```python
from build123d import *

# Parameters (mm, degrees)
SKETCH1_R           = 8.5
BOSS_EXTRUDE1_DEPTH = 1.9
BOSS_EXTRUDE2_DEPTH = 1.9
CIRPATTERN2_COUNT   = 12
FILLET5_R           = 6
FILLET6_R           = 6
BOSS_EXTRUDE3_DEPTH = 1.9
SKETCH6_W           = 11.017873235
SKETCH6_H           = 24.192230011
CUT_EXTRUDE2_DEPTH  = 24.342236397
SKETCH8_R           = 5
BOSS_EXTRUDE4_DEPTH = 3
SKETCH14_W          = 5
SKETCH14_H          = 10
BOSS_EXTRUDE8_DEPTH = 3
SKETCH17_R          = 1.5
CUT_EXTRUDE10_DEPTH = 24.342236397
FILLET9_R           = 2.5
FILLET10_R          = 2.5
CUT_EXTRUDE11_DEPTH = 2
SKETCH20_R          = 3.6
CUT_EXTRUDE12_DEPTH = 24.457408211


# Some blends are built 0.0001 mm under size
with BuildPart() as part:
    # Sketch1 → Boss-Extrude1 (new body)
    with BuildSketch(Plane.XY):
        with Locations(Location((0, 0, 0), (0, 0, 180))):
            Circle(SKETCH1_R)
    extrude(amount=BOSS_EXTRUDE1_DEPTH)

    # Sketch3 → Boss-Extrude2 (add)
    with BuildSketch(Plane.XY.offset(1.9)):
        Polygon((-1.305261922, 9.914448614), (-1.509060022, 7), (1.509060022, 7), (1.305261922, 9.914448614), (0.678518537, 11), (-0.678518537, 11), align=None)
    boss_extrude2 = extrude(amount=-BOSS_EXTRUDE2_DEPTH)

    # CirPattern2: Boss-Extrude2 ×12 about axis
    cirpattern2_axis = Axis((0, 0, 0), (0, 0, 1))
    for i in range(1, CIRPATTERN2_COUNT):
        add(boss_extrude2.rotate(cirpattern2_axis, i * 360 / CIRPATTERN2_COUNT))

    # Fillet5
    # the kernel refuses this fillet: 6 mm, written as the material it takes off along each edge
    with BuildSketch(Plane(origin=(9.238795325, 3.826834324, 5.354382408), x_dir=(0.49999999999981276, 0.8660254037845467, 0), z_dir=(0, 0, -1)), Plane(origin=(1.305261922, 9.914448614, 5.354382408), x_dir=(-0.5000000000001841, 0.8660254037843323, 0), z_dir=(0, 0, -1)), Plane(origin=(-7.933533403, 6.08761429, 5.354382408), x_dir=(-1, 0, 0), z_dir=(0, 0, -1)), Plane(origin=(-9.914448614, 1.305261922, 5.354382408), x_dir=(-0.8660254037843321, -0.5000000000001844, 0), z_dir=(0, 0, -1)), Plane(origin=(-9.238795325, -3.826834324, 5.354382408), x_dir=(-0.49999999999981826, -0.8660254037845436, 0), z_dir=(0, 0, -1)), Plane(origin=(-6.08761429, -7.933533403, 5.354382408), x_dir=(0, -1, 0), z_dir=(0, 0, -1)), Plane(origin=(3.826834324, -9.238795325, 5.354382408), x_dir=(0.8660254037845474, -0.49999999999981154, 0), z_dir=(0, 0, -1)), Plane(origin=(7.933533403, -6.08761429, 5.354382408), x_dir=(1, 0, 0), z_dir=(0, 0, -1)), Plane(origin=(9.914448614, -1.305261922, 5.354382408), x_dir=(0.866025403784333, 0.500000000000183, 0), z_dir=(0, 0, -1))) as fillet5_piece_1:
        with BuildLine():
            CenterArc((1.388315544, -5.998484909), FILLET5_R, 91.287628333, 24.712371667)
            Line((-1.241911337, -0.605720631), (-1.294515874, -0.497865346))
            Line((-1.294515874, -0.497865346), (-0.052604538, 0.107855286))
            Line((-0.052604538, 0.107855286), (0, 0.12))
            ThreePointArc((0, 0.12), (0.626743385, 0.12), (1.250790195, 0.119969698))
            Line((1.250790195, 0.119969698), (1.25348677, 0))
        make_face()
    extrude(amount=8.808764816, mode=Mode.SUBTRACT)
    with BuildSketch(Plane(origin=(6.08761429, 7.933533403, 5.354382408), x_dir=(-0.4383711467890806, -0.8987940462991654, 0), z_dir=(0, 0, -1)), Plane(origin=(-3.826834324, 9.238795325, 5.354382408), x_dir=(0.5591929034707432, -0.8290375725550441, 0), z_dir=(0, 0, -1)), Plane(origin=(-1.305261922, -9.914448614, 5.354382408), x_dir=(-0.06975647374412203, 0.9975640502598244, 0), z_dir=(0, 0, -1))) as fillet5_piece_2:
        with BuildLine():
            CenterArc((1.381752963, 6), FILLET5_R, 245.287628333, 24.712371667)
            Line((-1.126626446, 0.549492433), (-1.176794034, 0.440482282))
            ThreePointArc((-1.176794034, 0.440482282), (-0.615917761, 0.166890931), (-0.052604538, -0.107855286))
            Line((-0.052604538, -0.107855286), (0, -0.12))
            Line((0, -0.12), (1.381752963, -0.12))
            Line((1.381752963, -0.12), (1.381752963, 0))
        make_face()
    extrude(amount=8.808764816, mode=Mode.SUBTRACT)

    # Fillet6
    # the kernel refuses this fillet: 6 mm, written as the material it takes off along each edge
    with BuildSketch(Plane(origin=(7.933533403, 6.08761429, 5.354382408), x_dir=(-0.8987940462991681, -0.4383711467890751, 0), z_dir=(0, 0, -1)), Plane(origin=(3.826834324, 9.238795325, 5.354382408), x_dir=(-0.5591929034707512, -0.8290375725550386, 0), z_dir=(0, 0, -1)), Plane(origin=(-1.305261922, 9.914448614, 5.354382408), x_dir=(-0.06975647374412959, -0.9975640502598239, 0), z_dir=(0, 0, -1)), Plane(origin=(-6.08761429, 7.933533403, 5.354382408), x_dir=(0.43837114678907496, -0.8987940462991681, 0), z_dir=(0, 0, -1)), Plane(origin=(-9.238795325, 3.826834324, 5.354382408), x_dir=(0.8290375725550395, -0.5591929034707501, 0), z_dir=(0, 0, -1)), Plane(origin=(-9.914448614, -1.305261922, 5.354382408), x_dir=(0.9975640502598241, -0.0697564737441288, 0), z_dir=(0, 0, -1)), Plane(origin=(-7.933533403, -6.08761429, 5.354382408), x_dir=(0.8987940462991686, 0.4383711467890744, 0), z_dir=(0, 0, -1)), Plane(origin=(-3.826834324, -9.238795325, 5.354382408), x_dir=(0.5591929034707488, 0.8290375725550403, 0), z_dir=(0, 0, -1)), Plane(origin=(1.305261922, -9.914448614, 5.354382408), x_dir=(0.06975647374412966, 0.9975640502598239, 0), z_dir=(0, 0, -1)), Plane(origin=(6.08761429, -7.933533403, 5.354382408), x_dir=(-0.4383711467890749, 0.8987940462991683, 0), z_dir=(0, 0, -1)), Plane(origin=(9.238795325, -3.826834324, 5.354382408), x_dir=(-0.8290375725550393, 0.5591929034707505, 0), z_dir=(0, 0, -1)), Plane(origin=(9.914448614, 1.305261922, 5.354382408), x_dir=(-0.9975640502598239, 0.06975647374412894, 0), z_dir=(0, 0, -1))) as fillet6_piece_1:
        with BuildLine():
            CenterArc((1.381752963, -6), FILLET6_R, 90, 24.712371667)
            Line((-1.126626446, -0.549492433), (-1.176794034, -0.440482282))
            ThreePointArc((-1.176794034, -0.440482282), (-0.615917761, -0.166890931), (-0.052604538, 0.107855286))
            Line((-0.052604538, 0.107855286), (0, 0.12))
            Line((0, 0.12), (1.381752963, 0.12))
            Line((1.381752963, 0.12), (1.381752963, 0))
        make_face()
    extrude(amount=8.808764816, mode=Mode.SUBTRACT)

    # Sketch4 → Boss-Extrude3 (add)
    with BuildSketch(Plane(origin=(0, 0, 0), x_dir=(-1, 0, 0), z_dir=(0, 0, -1))):
        with BuildLine():
            Line((-2.5, 20.5), (-2.5, 4.330127019))
            ThreePointArc((-2.5, 4.330127019), (-5, 0), (-2.5, -4.330127019))
            Line((-2.5, -4.330127019), (-2.5, -11))
            Line((-2.5, -11), (2.5, -11))
            Line((2.5, -11), (2.5, -4.330127019))
            ThreePointArc((2.5, -4.330127019), (5, 0), (2.5, 4.330127019))
            Line((2.5, 4.330127019), (2.5, 20.5))
            Line((2.5, 20.5), (-2.5, 20.5))
        make_face()
    extrude(amount=-BOSS_EXTRUDE3_DEPTH)

    # Sketch6 → Cut-Extrude2 (cut, through all)
    with BuildSketch(Plane(origin=(0, 0, 0), x_dir=(-1, 0, 0), z_dir=(0, 0, -1))):
        with Locations((-8.008936618, 1.096115006)):
            Rectangle(SKETCH6_W, SKETCH6_H)
    extrude(amount=-CUT_EXTRUDE2_DEPTH, mode=Mode.SUBTRACT)

    # Sketch8 → Boss-Extrude4 (add)
    with BuildSketch(Plane(origin=(0, 0, 0), x_dir=(-1, 0, 0), z_dir=(0, 0, -1))):
        Circle(SKETCH8_R)
    extrude(amount=-BOSS_EXTRUDE4_DEPTH)

    # Sketch14 → Boss-Extrude8 (add)
    with BuildSketch(Plane(origin=(0, 0, 0), x_dir=(-1, 0, 0), z_dir=(0, 0, -1))):
        with Locations((2.5, 0)):
            Rectangle(SKETCH14_W, SKETCH14_H)
    extrude(amount=-BOSS_EXTRUDE8_DEPTH)

    # Sketch17 → Cut-Extrude10 (cut, through all)
    with BuildSketch(Plane.XY.offset(1.9)):
        with Locations((0, 18)):
            Circle(SKETCH17_R)
    extrude(amount=-CUT_EXTRUDE10_DEPTH, mode=Mode.SUBTRACT)

    # Fillet9
    fillet9_edges = [part.edges().sort_by_distance(p)[0] for p in [
        (-2.5, 20.5, 0.95),
        (2.5, 20.5, 0.95),
    ]]
    fillet(fillet9_edges, radius=FILLET9_R - 0.0001)  # a hair under: the kernel refuses the full size

    # Fillet10
    fillet10_edges = [part.edges().sort_by_distance(p)[0] for p in [
        (2.5, -11, 0.95),
    ]]
    fillet(fillet10_edges, radius=FILLET10_R)

    # Sketch19 → Cut-Extrude11 (cut)
    with BuildSketch(Plane.XY.offset(3)):
        Polygon((0, 3.6), (-5.102940329, 2.6), (-5.102940329, -2.6), (0, -3.6), align=None)
    extrude(amount=-CUT_EXTRUDE11_DEPTH, mode=Mode.SUBTRACT)

    # Sketch20 → Cut-Extrude12 (cut, through all)
    with BuildSketch(Plane.XY.offset(3)):
        Circle(SKETCH20_R)
    extrude(amount=-CUT_EXTRUDE12_DEPTH, mode=Mode.SUBTRACT)


solid = part.part
```
Geometry check sheet. Reference: the model listing, model coordinates, mm. A direction names the side the tool comes from. Round coordinates to 2 decimals unless told otherwise and drop trailing zeros. Order: outer loops, then holes, each group sorted by start corner. A loop starts at its lowest first (then second) coordinate and runs counter-clockwise, first axis right, second up. Notation, with made-up numbers: M 27,-7.75 L 35,-7.75 A21 ccw 35,15.25 Z; hole C -29,55 d6. An arc over 180 degrees is marked long. Write item = value, one per line.
Q1. Section check C-C (z = 0.6). Give the number of separate pieces and of enclosed holes in the cut face, plus the area to 3 significant figures.
Answer block:
separate_pieces = 1
enclosed_holes = 2
area = 222 mm^2
Q2. Section check D-D (x = -4.5). Enter the section's corners in (y, z).
Answer block:
outline = M -9.59,0 L 9.59,0 L 9.59,1.9 L 5,1.9 L 5,3 L 2.72,3 L 2.72,1 L -2.72,1 L -2.72,3 L -5,3 L -5,1.9 L -9.59,1.9 Z
Q3. Scan lines: line 1 (Y direction, x = 0, z = 0.95); line 2 (X direction, y = 0, z = 0.75); line 3 (Z direction, x = 0.5, y = 9.5). Record each from-to range of solid material in increasing order.
Answer block:
line_1 = -11 to -3.6, 3.6 to 16.5, 19.5 to 20.5
line_2 = -11 to -3.6, 3.6 to 5
line_3 = 0 to 1.9
Q4. Set-up check for faces 4 (the cylindrical face through (-3.9, 9.09, 0.96)), 5 (the cylindrical face through (-7.889, -5.916, 0.963)), 6 (the cylindrical face through (-5.924, -7.924, 0.963)): record each of +Z, -Z, +X, -X, +Y, -Y from which the full face is reachable in a straight line by a thin tool's end or side.
Answer block:
face_4 = +Z, -Z, +Y
face_5 = +Z, -Z, -Y
face_6 = +Z, -Z, -X
Q5. Release check for a two-part mould opening along Y. For faces 1 (the flat face through (-2.5, -10, 1)), 2 (the flat face through (-5.51, -9.52, 0.96)), 3 (the cylindrical face through (-6, 6.02, 0.94)) record: released by +Y, released by -Y, zero draft, split by the parting line, or undercut.
Answer block:
face_1 = zero draft
face_2 = released by -Y
face_3 = undercut
Q6. Section check A-A (x = 1). Enter the section's corners in (y, z), plus the area to 3 significant figures.
Answer block:
outline = M -10.79,0 L -3.46,0 L -3.46,3 L -4.9,3 L -4.9,1.9 L -10.79,1.9 Z; M 3.46,0 L 16.88,0 L 16.88,1.9 L 4.9,1.9 L 4.9,3 L 3.46,3 Z; M 19.12,0 L 20.29,0 L 20.29,1.9 L 19.12,1.9 Z
area = 44.8 mm^2
Q7. Section check B-B (y = 0). Enter the section's corners in (x, z), plus the area to 3 significant figures.
Answer block:
outline = M -11,0 L -3.6,0 L -3.6,1 L -5.1,1 L -5.1,1.9 L -11,1.9 Z; M 3.6,0 L 5,0 L 5,3 L 3.6,3 Z
area = 16.9 mm^2
Q8. Depth check by flat-ended pin: pin 1 Ø1.9 at (x, y) = (-3.5, -0.5) entering from +Z; pin 2 Ø0.9 at (y, z) = (-4.5, 2.5) entering from -X; pin 3 Ø1 at (x, z) = (2.5, 2) entering from +Y; pin 4 Ø4 at (x, y) = (0.5, -2) entering from -Z. Enter the tip coordinate at first touch or a pass-through.
Answer block:
pin_1 = 1
pin_2 = -5
pin_3 = 19.49
pin_4 = 0
